Check sheet for the modelled part. Datum: model origin and axes. Units: mm. A direction names the side the tool comes from. Coordinates: 2 decimals unless noted, no trailing zeros. Loops run counter-clockwise (first coordinate to the right, second up) from the corner with the lowest first, then second, coordinate; pieces in that order, holes last. Notation, with made-up numbers: (-19, 77.5) - (28, 77.5) arc R19 ccw to (28, 103.5) - close; hole circle Ø1 at (26.25, 86). An arc over 180 degrees is marked (long way). Use a Markdown table: item, result. Add a question column.
1) Sectioned sample at B-B, the plane z = 23.5. Enter the section's corners in (x, y), then the cut area to 3 significant figures.
2) Sectioned sample at C-C, the plane x = -9.5. Enter the section's corners in (y, z), then the cut area to 3 significant figures.
3) Thickness scan on line 1 (Z direction, x = 19.5, y = 11); line 2 (X direction, y = 13, z = 23); line 3 (Y direction, x = -22.5, z = -17). Record the ranges inside material, lowest first.
4) Go/stop test with flat-tipped pins: P1, Ø3, axis at y = 17, z = 14.5, coming from the +X side; P2, Ø15.5, axis at x = 29, y = 20.5, coming from the -Z side (3 decimals); P3, Ø0.8, axis at x = -11.5, y = 17.5, coming from the -Z side. Record where each tip stops, or that it passes through.
5) Sectioned sample at D-D, the plane x = 21.5. Enter the section's corners in (y, z) (3 decimals), then the cut area to 3 significant figures.
6) Tool access check on faces 5 (the cylindrical face through (-0.48, 13.82, -10.37)), 6 (the flat face through (27.1, 9.362, 27.127)), 7 (the flat face through (27, 24, 27.965)), 8 (the cylindrical face through (35.2, 26.1, -2.4)). Record the directions out of +Z, -Z, +X, -X, +Y, -Y that give a thin tool (end or side, any length) a straight path to the whole face; none if there is none.
7) Sectioned sample at A-A, the plane y = 15. Enter the section's corners in (x, z) (1 decimal), then the cut area to 3 significant figures.
8) Draft check along Z on faces 1 (the flat face through (27.1, 39.088, 27.127)), 2 (the flat face through (0, 40, -28)), 3 (the flat face through (0, 10, -12.75)), 4 (the flat face through (39.44, 31, 0)). Enter one of: pulls with the +Z half, pulls with the -Z half, needs draft (parallel to the pull), parting line crosses it, or undercut.
from build123d import *

# Parameters (mm, degrees)
SKETCH1_W               = 34
SKETCH1_H               = 19
BOSS_EXTRUDE1_DEPTH     = 20.2
SKETCH2_OUTSIDE_W       = 47.224
SKETCH2_OUTSIDE_H       = 32.224
SKETCH2_OUTSIDE_W_2     = 32.9
SKETCH2_OUTSIDE_H_2     = 18.5
CUT_EXTRUDE2_DEPTH      = 44.462627624
CUT_EXTRUDE8_DEPTH      = 36.679686097
CUT_EXTRUDE8_DEPTH_BACK = 36.679686097
SKETCH3_W               = 0.125
SKETCH3_H               = 9
CUT_EXTRUDE3_DEPTH      = 23.6
CHAMFER1_SIZE           = 1
CHAMFER2_SIZE           = 1
CHAMFER3_SIZE           = 1
CHAMFER4_SIZE           = 1
SKETCH10_R              = 3
BOSS_EXTRUDE3_DEPTH     = 3
FILLET1_R               = 2
SCALE_1_SCALE           = 1.7


with BuildPart() as part:
    # Sketch1 → Boss-Extrude1 (new, symmetric)
    with BuildSketch(Plane(origin=(0, 0, 0), x_dir=(0, 0, -1), z_dir=(1, 0, 0))):
        with Locations((0, 14.5)):
            Rectangle(SKETCH1_W, SKETCH1_H)
    extrude(amount=BOSS_EXTRUDE1_DEPTH, both=True)

    # Sketch2 outside → Cut-Extrude2 (cut, through all)
    with BuildSketch(Plane(origin=(11.8, 0, 0), x_dir=(0, 0, -1), z_dir=(1, 0, 0))):
        with Locations((0, 14.5)):
            Rectangle(SKETCH2_OUTSIDE_W, SKETCH2_OUTSIDE_H)
        with Locations((0, 14.25)):
            Rectangle(SKETCH2_OUTSIDE_W_2, SKETCH2_OUTSIDE_H_2, mode=Mode.SUBTRACT)
    cut_extrude2 = extrude(amount=CUT_EXTRUDE2_DEPTH, mode=Mode.SUBTRACT)

    # Mirror1: Cut-Extrude2 across plane
    add(cut_extrude2.mirror(Plane(origin=(0, 0, 0), x_dir=(0, 0, 1), z_dir=(1, 0, 0))), mode=Mode.SUBTRACT)

    # Sketch5 → Cut-Extrude8 (cut, two sides: drawn at the far end of the back side and taken through both)
    with BuildSketch(Plane(origin=(0, 0, 0), x_dir=(0, 0, -1), z_dir=(1, 0, 0)).offset(-CUT_EXTRUDE8_DEPTH_BACK)):
        with BuildLine():
            Line((-5.692330317, 12.5), (5.692330317, 12.5))
            Line((5.692330317, 12.5), (6.192330317, 12))
            ThreePointArc((6.192330317, 12), (6.706274607, 11.346743741), (7.5, 11.1))
            Line((7.5, 11.1), (7.5, 9.5))
            ThreePointArc((7.5, 9.5), (6.1, 8.1), (7.5, 6.7))
            Line((7.5, 6.7), (7.5, 1))
            Line((7.5, 1), (6.5, 0))
            Line((6.5, 0), (-6.5, 0))
            Line((-6.5, 0), (-7.5, 1))
            Line((-7.5, 1), (-7.5, 6.7))
            ThreePointArc((-7.5, 6.7), (-6.1, 8.1), (-7.5, 9.5))
            Line((-7.5, 9.5), (-7.5, 11.1))
            ThreePointArc((-7.5, 11.1), (-6.706274607, 11.346743741), (-6.192330317, 12))
            Line((-6.192330317, 12), (-5.692330317, 12.5))
        make_face()
    extrude(amount=CUT_EXTRUDE8_DEPTH + CUT_EXTRUDE8_DEPTH_BACK, mode=Mode.SUBTRACT)

    # Sketch3 → Cut-Extrude3 (cut)
    with BuildSketch(Plane(origin=(11.8, 0, 0), x_dir=(0, 0, -1), z_dir=(1, 0, 0))):
        with Locations((-16.9375, 9.5)):
            Rectangle(SKETCH3_W, SKETCH3_H)
    cut_extrude3 = extrude(amount=-CUT_EXTRUDE3_DEPTH, mode=Mode.SUBTRACT)

    # Mirror2: Cut-Extrude3 across plane
    add(cut_extrude3.mirror(Plane.XY), mode=Mode.SUBTRACT)

    # Chamfer1
    chamfer1_edges = [part.edges().sort_by_distance(p)[0] for p in [
        (16, 23.5, -16.45),
        (16, 23.5, 16.45),
        (-16, 23.5, 16.45),
        (-16, 23.5, -16.45),
    ]]
    chamfer(chamfer1_edges, length=CHAMFER1_SIZE)

    # Chamfer2
    chamfer2_edges = [part.edges().sort_by_distance(p)[0] for p in [
        (0, 24, 17),
        (0, 24, -17),
    ]]
    chamfer(chamfer2_edges, length=CHAMFER2_SIZE)

    # Chamfer3
    chamfer3_edges = [part.edges().sort_by_distance(p)[0] for p in [
        (16, 5, 16.45),
        (16, 5, -16.45),
        (-16, 5, -16.45),
        (-16, 5, 16.45),
    ]]
    chamfer(chamfer3_edges, length=CHAMFER3_SIZE)

    # Chamfer4
    chamfer4_edges = [part.edges().sort_by_distance(p)[0] for p in [
        (0, 5, 16.875),
        (0, 5, -16.875),
    ]]
    chamfer(chamfer4_edges, length=CHAMFER4_SIZE)

    # Sketch10 → Boss-Extrude3 (add)
    with BuildSketch(Plane(origin=(20.2, 0, 0), x_dir=(0, 0, -1), z_dir=(1, 0, 0))):
        with Locations((0, 18)):
            Circle(SKETCH10_R)
    extrude(amount=BOSS_EXTRUDE3_DEPTH)

    # Fillet1
    fillet1_edges = [part.edges().sort_by_distance(p)[0] for p in [
        (23.2, 18, 3),
    ]]
    fillet(fillet1_edges, radius=FILLET1_R)


with BuildPart() as part_1:
    # Scale 1: scaled about (0, 0, 0)
    add(part.part.scale(SCALE_1_SCALE))


solid = part_1.part
Solved:
| question | item | result |
|---|---|---|
| 1 | outline | (-34.34, 8.5) - (34.34, 8.5) - (34.34, 39.95) - (20.06, 39.95) - (20.06, 40.8) - (-20.06, 40.8) - (-20.06, 39.95) - (-34.34, 39.95) - close |
| 1 | area | 2,190 mm2 |
| 2 | outline | (8.5, -26.99) - (10.2, -28.69) - (23.8, -28.69) - (23.8, -28.9) - (39.1, -28.9) - (40.8, -27.2) - (40.8, 27.2) - (39.1, 28.9) - (23.8, 28.9) - (23.8, 28.69) - (10.2, 28.69) - (8.5, 26.99) - (8.5, 12.75) - (11.39, 12.75) arc R2.38 ccw to (16.15, 12.75) - (18.87, 12.75) arc R2.38 ccw to (20.4, 10.53) - (21.25, 9.68) - (21.25, -9.68) - (20.4, -10.53) arc R2.38 ccw to (18.87, -12.75) - (16.15, -12.75) arc R2.38 ccw to (11.39, -12.75) - (8.5, -12.75) - close |
| 2 | area | 1,560 mm2 |
| 3 | line 1 | z = -28.69 to -12.75, 12.75 to 28.69 |
| 3 | line 2 | x = -34.34 to 34.34 |
| 3 | line 3 | y = 8.5 to 39.95 |
| 4 | P1 | stops at x = 34.34 |
| 4 | P2 | stops at z = -27.965 |
| 4 | P3 | stops at z = -28.69 |
| 5 | outline | (8.5, -26.265) - (10.2, -27.965) - (38.25, -27.965) - (39.95, -26.265) - (39.95, 26.265) - (38.25, 27.965) - (10.2, 27.965) - (8.5, 26.265) - (8.5, 12.75) - (11.39, 12.75) arc R2.38 ccw to (16.15, 12.75) - (18.87, 12.75) arc R2.38 ccw to (20.4, 10.527) - (21.25, 9.677) - (21.25, -9.677) - (20.4, -10.527) arc R2.38 ccw to (18.87, -12.75) - (16.15, -12.75) arc R2.38 ccw to (11.39, -12.75) - (8.5, -12.75) - close |
| 5 | area | 1,460 mm2 |
| 6 | face 5 | +X, -X |
| 6 | face 6 | +Z, +X, -Y |
| 6 | face 7 | +Z, +X, +Y, -Y |
| 6 | face 8 | +X |
| 7 | outline | (-34.3, -28) - (-20.1, -28) - (-20.1, -28.7) - (20.1, -28.7) - (20.1, -28) - (34.3, -28) - (34.3, -10.7) - (-34.3, -10.7) - close; (-34.3, 10.7) - (34.3, 10.7) - (34.3, 28) - (20.1, 28) - (20.1, 28.7) - (-20.1, 28.7) - (-20.1, 28) - (-34.3, 28) - close |
| 7 | area | 2,430 mm2 |
| 8 | face 1 | pulls with the +Z half |
| 8 | face 2 | pulls with the -Z half |
| 8 | face 3 | undercut |
| 8 | face 4 | needs draft |
